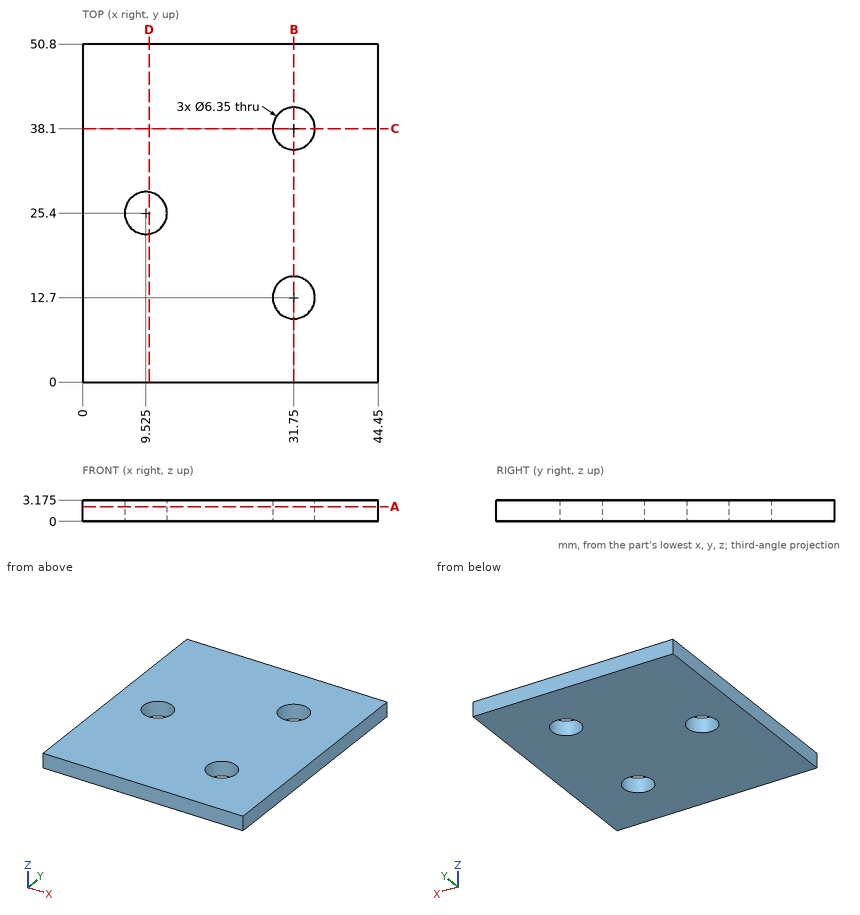
Drawing for the job (mm, zero at the part's lowest x, y, z). Coordinates: 2 decimals unless noted, no trailing zeros. Write each loop counter-clockwise with the first axis right and the second up, starting at its lowest first coordinate (ties: lowest second). Pieces come first, ordered by that corner, then holes. Notation, with made-up numbers: (-12, 66) - (35, 66) arc R25 ccw to (35, 80) - close; hole circle Ø1 at (-11, 4.25). An arc over 180 degrees is marked (long way). Write each question's results on one line, items separated by ' | '. Start each with the question number.
1) Probe line 1 along Y through (x, z) = (31.75, 1.65) (3 decimals); line 2 along Y through (x, z) = (34.5, 1.9); line 3 along Y through (x, z) = (8, 0.45). List the from-to ranges inside material, lowest first. Write a range as from..to.
2) Flat gauge pin, fed straight in: P1, Ø7.5, axis at x = 9.525, y = 25.4, coming from the -Z side. Where does the tip first touch, or does it go through?
3) Cut at D-D (x = 10). Write the cut outline in (y, z) (3 decimals).
4) Cut at B-B (x = 31.75). Write the cut outline in (y, z) (3 decimals), then the cut area to 3 significant figures.
5) Cut at C-C (y = 38.1). Write the cut outline in (x, z) (3 decimals), then the cut area to 3 significant figures.
6) Cut at A-A (z = 2.2). Write the cut outline in (x, y) (3 decimals), then the cut area to 3 significant figures.
Returned:
1) line 1: 0..9.525, 15.875..34.925, 41.275..50.8 | line 2: 0..11.11, 14.29..36.51, 39.69..50.8 | line 3: 0..22.62, 28.18..50.8
2) P1: z = 0
3) outline: (0, 0) - (22.261, 0) - (22.261, 3.175) - (0, 3.175) - close; (28.539, 0) - (50.8, 0) - (50.8, 3.175) - (28.539, 3.175) - close
4) outline: (0, 0) - (9.525, 0) - (9.525, 3.175) - (0, 3.175) - close; (15.875, 0) - (34.925, 0) - (34.925, 3.175) - (15.875, 3.175) - close; (41.275, 0) - (50.8, 0) - (50.8, 3.175) - (41.275, 3.175) - close | area: 121 mm^2
5) outline: (0, 0) - (28.575, 0) - (28.575, 3.175) - (0, 3.175) - close; (34.925, 0) - (44.45, 0) - (44.45, 3.175) - (34.925, 3.175) - close | area: 121 mm^2
6) outline: (0, 0) - (44.45, 0) - (44.45, 50.8) - (0, 50.8) - close; hole circle Ø6.35 at (9.525, 25.4); hole circle Ø6.35 at (31.75, 12.7); hole circle Ø6.35 at (31.75, 38.1) | area: 2,160 mm^2
